Geometry: final body of the model. Coordinates: model frame, mm. Face numbers are marked on the shaded views. A direction names the side the tool comes from. Round coordinates to 2 decimals unless told otherwise and drop trailing zeros. Loops run counter-clockwise (first coordinate to the right, second up) from the corner with the lowest first, then second, coordinate; pieces in that order, holes last. Notation, with made-up numbers: (-32.5, 52.5) - (-17.5, 52.5) arc R14 ccw to (-17.5, 59.5) - close; hole circle Ø1 at (-36, 54). An arc over 180 degrees is marked (long way). Answer as CSV lines item,"result".
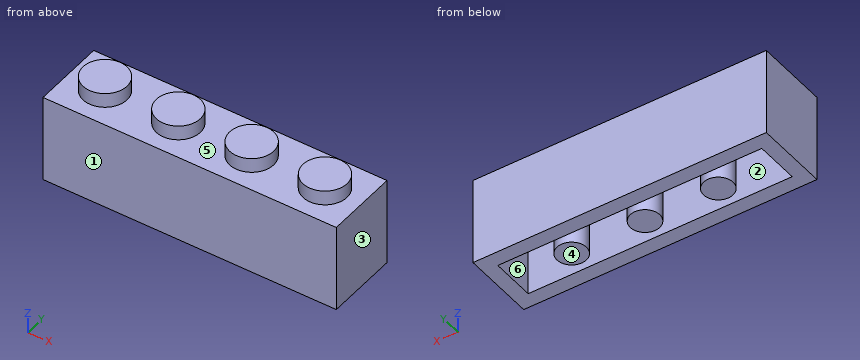
from build123d import *

# Parameters (mm, degrees)
SKETCH1_W           = 32
SKETCH1_H           = 8
BOSS_EXTRUDE1_DEPTH = 9.6
SKETCH2_R           = 2.4
BOSS_EXTRUDE2_DEPTH = 1.6
LPATTERN1_COUNT     = 4
LPATTERN1_PITCH     = 8
SHELL1_T            = -1.6
SKETCH3_R           = 1.6
BOSS_EXTRUDE3_DEPTH = 8
LPATTERN2_COUNT     = 3
LPATTERN2_PITCH     = 8


with BuildPart() as part:
    # Sketch1 → Boss-Extrude1 (new body)
    with BuildSketch(Plane.XY):
        with Locations((16, 4)):
            Rectangle(SKETCH1_W, SKETCH1_H)
    extrude(amount=BOSS_EXTRUDE1_DEPTH)

    # Sketch2 → Boss-Extrude2 (add)
    with BuildSketch(Plane.XY.offset(9.6)):
        with Locations((4, 4)):
            Circle(SKETCH2_R)
    boss_extrude2 = extrude(amount=BOSS_EXTRUDE2_DEPTH)

    # LPattern1: Boss-Extrude2 ×4
    with Locations(*[(i * LPATTERN1_PITCH, 0, 0) for i in range(1, LPATTERN1_COUNT)]):
        add(boss_extrude2)

    # Shell1
    shell1_openings = [part.faces().sort_by_distance(p)[0] for p in [
        (16, 4, 0),
    ]]
    offset(amount=SHELL1_T, openings=shell1_openings, kind=Kind.INTERSECTION)

    # Sketch3 → Boss-Extrude3 (add)
    with BuildSketch(Plane(origin=(0, 0, 8), x_dir=(-1, 0, 0), z_dir=(0, 0, -1))):
        with Locations((-8, 4)):
            Circle(SKETCH3_R)
    boss_extrude3 = extrude(amount=BOSS_EXTRUDE3_DEPTH)

    # LPattern2: Boss-Extrude3 ×3
    with Locations(*[(i * LPATTERN2_PITCH, 0, 0) for i in range(1, LPATTERN2_COUNT)]):
        add(boss_extrude3)


solid = part.part
(1) Section C-C (x = 16). Output: boundary loops of the cut face in (y, z), and give its area (3 significant figures).
Findings below:
outline,"(0, 0) - (1.6, 0) - (1.6, 8) - (2.4, 8) - (2.4, 0) - (5.6, 0) - (5.6, 8) - (6.4, 8) - (6.4, 0) - (8, 0) - (8, 9.6) - (0, 9.6) - close"
area,"64.0 mm2"
(2) Section D-D (y = 0.5). Output: boundary loops of the cut face in (x, z).
Findings below:
outline,"(0, 0) - (32, 0) - (32, 9.6) - (0, 9.6) - close"
(3) Access query for the marked faces 4, 5 and 6. Directions: +Z, -Z, +X, -X, +Y, -Y. A direction counts if a zero-diameter tool reaches every point of the face in a straight line with its end or side. Return the directions, or none.
Findings below:
face 4,"-Z, +X, -X, +Y, -Y"
face 5,"+Z"
face 6,"-Z"
(4) Section A-A (z = 7). Output: boundary loops of the cut face in (x, y).
Findings below:
outline,"(0, 0) - (32, 0) - (32, 8) - (0, 8) - close; circle Ø3.2 at (8, 4); circle Ø3.2 at (16, 4); circle Ø3.2 at (24, 4); hole (1.6, 1.6) - (30.4, 1.6) - (30.4, 6.4) - (1.6, 6.4) - close"
(5) Draft query along X for the marked faces 1, 2 and 3. Return one class per face: pulls with the +X half, pulls with the -X half, needs draft (parallel to the pull), parting line crosses it, or undercut.
Findings below:
face 1,"needs draft"
face 2,"undercut"
face 3,"pulls with the +X half"
(6) Pin query (flat end, axial travel): P1, Ø0.5, axis at x = 4.5, y = 4, coming from the -Z side; P2, Ø1.8, axis at x = 19.5, y = 4, coming from the -Z side. Return the tip coordinate at first contact, or that it passes through.
Findings below:
P1,"z = 9.6"
P2,"z = 8"
(7) Section B-B (z = 9). Output: boundary loops of the cut face in (x, y).
Findings below:
outline,"(0, 0) - (32, 0) - (32, 8) - (0, 8) - close; hole circle Ø1.6 at (4, 4); hole circle Ø1.6 at (12, 4); hole circle Ø1.6 at (20, 4); hole circle Ø1.6 at (28, 4)"
(8) Material intervals for line 1 along X through (y, z) = (4, 8.65); line 2 along X through (y, z) = (3.25, 7); line 3 along Y through (x, z) = (20, 8.45), sorted ascending.
Findings below:
line 1,"0 to 3.2, 4.8 to 11.2, 12.8 to 19.2, 20.8 to 27.2, 28.8 to 32"
line 2,"0 to 1.6, 6.59 to 9.41, 14.59 to 17.41, 22.59 to 25.41, 30.4 to 32"
line 3,"0 to 3.2, 4.8 to 8"
